Check sheet for the modelled part. Datum: model origin and axes. Units: mm. Face numbers are marked on the shaded views. A direction names the side the tool comes from. Round coordinates to 2 decimals unless told otherwise and drop trailing zeros. Order: outer loops, then holes, each group sorted by start corner. A loop starts at its lowest first (then second) coordinate and runs counter-clockwise, first axis right, second up. Notation, with made-up numbers: (-2.5, 45) -> (43.5, 45) arc R34 cw to (43.5, 84) -> close; hole circle Ø11 at (20.5, 41.25). An arc over 180 degrees is marked (long way). Answer in a Markdown table with one row per item.
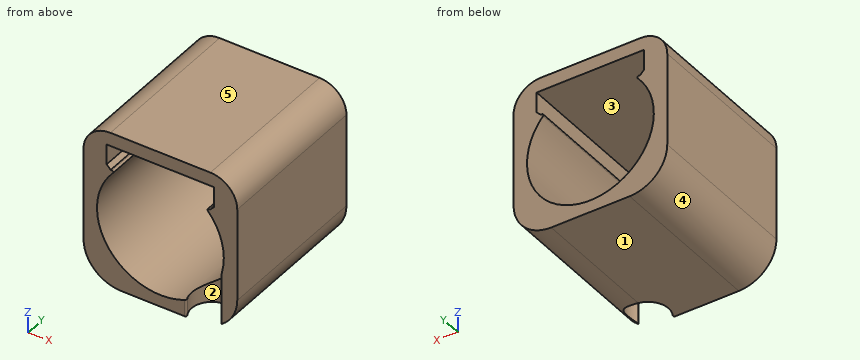
Autodesk Inventor part; units mm, degrees
ref_plane "YZ Plane" through (0, 0, 0) normal (1, 0, 0) x (0, 1, 0)
ref_plane "XZ Plane" through (0, 0, 0) normal (0, 1, 0) x (-1, 0, 0)
ref_plane "XY Plane" through (0, 0, 0) normal (0, 0, 1) x (1, 0, 0)
sketch "Sketch1" plane through (0, 0, 0) normal (0, 1, 0) x (-1, 0, 0)
  circle A0 centre (0, 0) radius 11.5
  circle A1 centre (0, 0) radius 11.8
  line L0 (10, 12.5) -> (-10, 12.5)
  line L1 (-10, 12.5) -> (-10, 8.2614)
  line L2 (-10, 8.2614) -> (10, 8.2614)
  line L3 (10, 8.2614) -> (10, 12.5)
  line L4 (10, 12.5) -> (-10, 8.2614) construction
  line L5 (-10, 12.5) -> (10, 8.2614) construction
  line L6 (0, 10.3807) -> (0, -11.5) construction
  line L7 (10, 12.5) -> (-10, 12.5)
  line L8 (-10, 12.5) -> (-10, 12.8)
  line L9 (-10, 12.8) -> (10, 12.8)
  line L10 (10, 12.8) -> (10, 12.5)
  line L11 (-14.3, 15.3) -> (14.3, 15.3)
  line L12 (14.3, 15.3) -> (14.3, -14)
  line L13 (14.3, -14) -> (-14.3, -14)
  line L14 (-14.3, -14) -> (-14.3, 15.3)
  point P0 (8, 8.2614)
  point P1 (-8, 8.2614)
  point P2 (0, -14)
  point P3 (8.4256, 8.2614)
  point P4 (-8.4256, 8.2614)
  dimension "d0" = 23
  dimension "d1" = 0.3
  dimension "d2" = 24
  dimension "d3" = 16
  dimension "d4" = 20
  dimension "d5" = 0.3
  dimension "d6" = 2.5
  dimension "d7" = 2.5
  dimension "d8" = 2.5
  dimension "d9" = 14.3
  dimension "d10" = 14.3
extrude "Extrusion1" add sketch "Sketch1" along normal blind 30
fillet "Fillet1" radius 0.25 2 edges at (8.4256, 15, 8.2614) (-8.4256, 15, 8.2614)
chamfer "Chamfer1" distance 0.75 angle 45 2 edges at (-10, 15, 8.2614) (10, 15, 8.2614)
sketch "Sketch2" plane through (14.3, 0, -14) normal (0, 0, -1) x (-1, 0, 0)
  line L0 (2.5, 30) -> (26.1, 30)
  line L1 (2.5, 30) -> (26.1, 30)
  line L2 (26.1, 30) -> (26.1, 0)
  line L3 (26.1, 0) -> (2.5, 0)
  line L4 (2.5, 0) -> (2.5, 30)
  line L5 (0, 0) -> (28.6, 0)
  circle A0 centre (6.3, 2.3324) radius 3.5
  circle A1 centre (6.3, 2.3324) radius 3.8
  line L6 (3.3, 0) -> (9.3, 0) construction
  line L7 (2.8, 0) -> (2.8, 30)
  point P0 (14.3, 0)
  point P1 (23.1144, 30)
  point P2 (5.4856, 30)
  point P3 (2.5, 2.3324)
  point P4 (3.6904, 0)
  point P5 (9.3, 0)
  point P6 (2.5, 2.3324)
  point P7 (2.5, 0.8525)
  point P8 (8.9096, 0)
  dimension "d17" = 7
  dimension "d18" = 0.3
  dimension "d20" = 6
  dimension "d25" = 0.3
extrude "Extrusion2" cut sketch "Sketch2" against normal up to surface contours A1 L7 | A1 L3 A0 L7 | L7 A0 L3 A1 | A0 L3 | L3 A0 A1 | L3 A0
fillet "Fillet2" radius 0.25 2 edges at (5, 0, -12.3442) (11, 0, -9.1354)
sketch "Sketch4" plane through (14.3, 30, -14) normal (0, 0, -1) x (-1, 0, 0)
  arc A0 (2.8264, -30) -> (3.0408, -29.6215) centre (2.8264, -29.75) ccw
  arc A1 (9.5592, -29.6215) -> (3.0408, -29.6215) centre (6.3, -27.6676) ccw
  arc A2 (9.5592, -29.6215) -> (9.7736, -30) centre (9.7736, -29.75) ccw
  line L0 (9.7736, -30) -> (28.6, -30)
  line L1 (28.6, -30) -> (28.6, 0)
  line L2 (0, 0) -> (28.6, 0)
  line L3 (0, -30) -> (0, 0)
  line L4 (0, -30) -> (2.8264, -30)
  line L5 (3.0764, -29.0955) -> (9.5236, -29.0955)
  line L6 (9.5236, -29.0955) -> (9.5236, -29.986)
  line L7 (9.5236, -29.986) -> (3.0764, -29.986)
  line L8 (3.0764, -29.986) -> (3.0764, -29.0955)
  arc A3 (9.5592, -29.6215) -> (9.7736, -30) centre (9.7736, -29.75) ccw
  point P0 (14.3, -30)
  dimension "d26" = 6.4473
fillet "Fillet3" radius 7 2 edges at (14.3, 15, -14) (-14.3, 15, -14)
fillet "Fillet4" radius 5 2 edges at (-14.3, 15, 15.3) (14.3, 15, 15.3)
sketch "Sketch5" plane through (0, 30, 0) normal (0, 1, 0) x (1, 0, 0)
  arc A0 (8.8144, -7.8451) -> (-8.8144, -7.8451) centre (0, 0) ccw
  line L0 (10, -12.8) -> (-10, -12.8)
  line L1 (-10, -12.8) -> (-10, -9.0114)
  line L2 (-9.25, -8.2614) -> (-10, -9.0114)
  line L3 (-9.25, -8.2614) -> (-9.0011, -8.2614)
  arc A1 (-9.0011, -8.2614) -> (-8.8144, -7.8451) centre (-9.0011, -8.0114) ccw
  line L4 (10, -9.0114) -> (10, -12.8)
  arc A2 (-9.0011, -8.2614) -> (-8.8144, -7.8451) centre (-9.0011, -8.0114) ccw
  arc A3 (8.8144, -7.8451) -> (-8.8144, -7.8451) centre (0, 0) ccw
  arc A4 (8.8144, -7.8451) -> (9.0011, -8.2614) centre (9.0011, -8.0114) ccw
  line L5 (9.0011, -8.2614) -> (9.25, -8.2614)
  line L6 (10, -9.0114) -> (9.25, -8.2614)
  line L7 (10, -9.0114) -> (10, -12.8)
  line L8 (10, -12.8) -> (-10, -12.8)
  line L9 (-10, -12.8) -> (-10, -9.0114)
  line L10 (-9.25, -8.2614) -> (-10, -9.0114)
  line L11 (-9.25, -8.2614) -> (-9.0011, -8.2614)
equation "\"d10\" = d9"
properties part number "mount"
Item 1: Mould release check, pull along X, two halves, no side actions. Record for the marked faces 3, 4 and 5: pulls with the +X half, pulls with the -X half, needs draft (parallel to the pull), parting line crosses it, or undercut.
Result sheet:
| item | result |
|---|---|
| face 3 | undercut |
| face 4 | pulls with the -X half |
| face 5 | needs draft |
Item 2: Cross-section at B-B (z = 9.5). Record the boundary of the cut face in (x, y).
Result sheet:
| item | result |
|---|---|
| outline | (-14.3, 0) -> (-10, 0) -> (-10, 30) -> (-14.3, 30) -> close; (10, 0) -> (14.3, 0) -> (14.3, 30) -> (10, 30) -> close |
Item 3: Cross-section at C-C (y = 22.5). Record the boundary of the cut face in (x, z), and give its area (3 significant figures).
Result sheet:
| item | result |
|---|---|
| outline | (-14.3, -7) arc R7 ccw to (-7.3, -14) -> (7.3, -14) arc R7 ccw to (14.3, -7) -> (14.3, 10.3) arc R5 ccw to (9.3, 15.3) -> (-9.3, 15.3) arc R5 ccw to (-14.3, 10.3) -> close; hole (-10, 9.01) -> (-9.25, 8.26) -> (-9, 8.26) arc R0.25 cw to (-8.81, 7.85) arc R11.8 ccw (long way) to (8.81, 7.85) arc R0.25 cw to (9, 8.26) -> (9.25, 8.26) -> (10, 9.01) -> (10, 12.8) -> (-10, 12.8) -> close |
| area | 320 mm^2 |
Item 4: Cross-section at A-A (x = 0). Record the boundary of the cut face in (y, z).
Result sheet:
| item | result |
|---|---|
| outline | (0, -14) -> (30, -14) -> (30, -11.8) -> (0, -11.8) -> close; (0, 12.8) -> (30, 12.8) -> (30, 15.3) -> (0, 15.3) -> close |
Item 5: Scan lines: line 1 (X direction, y = 20, z = 0); line 2 (Z direction, x = 0, y = 22.5); line 3 (X direction, y = 8, z = -7). Record each from-to range of solid material in increasing order. Write a range as [from, to].
Result sheet:
| item | result |
|---|---|
| line 1 | x = [-14.3, -11.8], [11.8, 14.3] |
| line 2 | z = [-14, -11.8], [12.8, 15.3] |
| line 3 | x = [-14.3, -9.5], [9.5, 14.3] |
Item 6: Set-up check for the marked faces 1 and 2: record each of +Z, -Z, +X, -X, +Y, -Y from which the full face is reachable in a straight line by a thin tool's end or side.
Result sheet:
| item | result |
|---|---|
| face 1 | -Z, +X, -X, +Y, -Y |
| face 2 | -Z |
Item 7: Depth check by flat-ended pin: P1, Ø1.5, axis at x = 10.5, y = 9, coming from the +Z side. Enter the tip coordinate at first touch or a pass-through.
Result sheet:
| item | result |
|---|---|
| P1 | stops at z = 15.28 |
